from build123d import *

# Parameters (mm, degrees)
F0_W       = 50.8
F0_H       = 31.75
F1_DEPTH   = 15.875
F2_W       = 38.1
F2_H       = 31.75
F3_DEPTH   = 6.35
F4_SIZE2   = 5.08
F4_SIZE    = 2.54
F4_2_SIZE2 = 5.08
F4_2_SIZE  = 2.54


with BuildPart() as f1:
    # F0 (on Top) → F1 (new body)
    with BuildSketch(Plane.XY):
        Rectangle(F0_W, F0_H)
    extrude(amount=-F1_DEPTH)

    # F2 (on face) → F3 (cut)
    with BuildSketch(Plane(origin=(0, 0, -15.875), x_dir=(1, 0, 0), z_dir=(0, 0, -1))):
        Rectangle(F2_W, F2_H)
    extrude(amount=-F3_DEPTH, mode=Mode.SUBTRACT)

    # F4
    f4_edges = [f1.edges().sort_by_distance(p)[0] for p in [
        (-25.4, 0, 0),
    ]]
    f4_side = f1.faces().sort_by_distance((-25.4, 0, -7.9375))[0]
    chamfer(f4_edges, length=F4_SIZE, length2=F4_SIZE2, reference=f4_side)

    # F4#2
    f4_2_edges = [f1.edges().sort_by_distance(p)[0] for p in [
        (25.4, 0, 0),
    ]]
    f4_2_side = f1.faces().sort_by_distance((25.4, 0, -7.9375))[0]
    chamfer(f4_2_edges, length=F4_2_SIZE, length2=F4_2_SIZE2, reference=f4_2_side)


solid = f1.part
Verification items for the finished model (mm, model axes). A direction names the side the tool comes from. Coordinates: 2 decimals unless noted, no trailing zeros. Order: outer loops, then holes, each group sorted by start corner. A loop starts at its lowest first (then second) coordinate and runs counter-clockwise, first axis right, second up.
1. Set-up check for faces 1 (the face through (0, 15.875, -6)), 2 (the face through (0, 0, -9.525)): record each of +Z, -Z, +X, -X, +Y, -Y from which the full face is reachable in a straight line by a thin tool's end or side.
Results found:
face 1: +Z, -Z, +X, -X, +Y
face 2: -Z, +Y, -Y
2. Sectioned sample at D-D, the plane x = -14.5. Record the cut outline in (y, z) (3 decimals).
Results found:
outline: (-15.875, -9.525) - (15.875, -9.525) - (15.875, 0) - (-15.875, 0) - close
3. Sectioned sample at A-A, the plane z = -12.5. Record the cut outline in (x, y) (3 decimals), and give its area (3 significant figures).
Results found:
outline: (-25.4, -15.875) - (-19.05, -15.875) - (-19.05, 15.875) - (-25.4, 15.875) - close; (19.05, -15.875) - (25.4, -15.875) - (25.4, 15.875) - (19.05, 15.875) - close
area: 403 mm2
4. Release check for a two-part mould opening along X. For faces 3 (the face through (-22.82, -0.22, -1.25)), 4 (the face through (-22, 0, -15.875)), 5 (the face through (-19.05, 0, -13)) record: +X half, -X half, draft (parallel to the pull), parting line (faces both ways), or undercut.
Results found:
face 3: -X half
face 4: draft
face 5: undercut
5. Go/stop test with a flat-tipped pin: pin 1 Ø9.5 at (x, y) = (-5, -6.5) entering from -Z (3 decimals). Record where the tip stops, or that it passes through.
Results found:
pin 1: stops at z = -9.525
6. Sectioned sample at C-C, the plane x = 21.5. Record the cut outline in (y, z) (3 decimals).
Results found:
outline: (-15.875, -15.875) - (15.875, -15.875) - (15.875, -0.59) - (-15.875, -0.59) - close
7. Scan lines: line 1 (X direction, y = 12.5, z = -14.75); line 2 (Z direction, x = 2, y = -8) (3 decimals); line 3 (X direction, y = -12, z = -2.5). Record each from-to range of solid material in increasing order.
Results found:
line 1: x = -25.4 to -19.05, 19.05 to 25.4
line 2: z = -9.525 to 0
line 3: x = -25.32 to 25.32
8. Sectioned sample at B-B, the plane y = 2.5. Record the cut outline in (x, z) (3 decimals), and give its area (3 significant figures).
Results found:
outline: (-25.4, -15.875) - (-19.05, -15.875) - (-19.05, -9.525) - (19.05, -9.525) - (19.05, -15.875) - (25.4, -15.875) - (25.4, -2.54) - (20.32, 0) - (-20.32, 0) - (-25.4, -2.54) - close
area: 552 mm2
